Build history of the part. All positions in model axes, mm. Face numbers are marked on the shaded views. A direction names the side the tool comes from. Round coordinates to 2 decimals unless told otherwise and drop trailing zeros. Write each loop counter-clockwise with the first axis right and the second up, starting at its lowest first coordinate (ties: lowest second). Pieces come first, ordered by that corner, then holes. Notation, with made-up numbers: (66, -6.75) -> (108, -6.75) arc R35 ccw to (108, 25.25) -> close; hole circle Ø9 at (81.25, 65). An arc over 180 degrees is marked (long way). Answer as CSV lines item,"result".
from build123d import *

# Parameters (mm, degrees)
SKETCH1_W           = 33
SKETCH1_H           = 33
SKETCH1_R           = 1.5
BOSS_EXTRUDE1_DEPTH = 2.5
FILLET1_R           = 5
SKETCH2_W           = 15
SKETCH2_H           = 5.6
SKETCH2_W_2         = 5.6
SKETCH2_H_2         = 15
BOSS_EXTRUDE2_DEPTH = 7
SKETCH3_W           = 12
SKETCH3_H           = 11
BOSS_EXTRUDE3_DEPTH = 4


with BuildPart() as part:
    # Sketch1 → Boss-Extrude1 (new body)
    with BuildSketch(Plane.XY):
        with Locations((-3.4417913, -5.340458015)):
            Rectangle(SKETCH1_W, SKETCH1_H)
        with Locations((-15.4417913, 6.659541985)):
            Circle(SKETCH1_R, mode=Mode.SUBTRACT)
        with Locations(Location((8.5582087, 6.659541985, 0), (0, 0, 180))):
            Circle(SKETCH1_R, mode=Mode.SUBTRACT)
        with Locations(Location((-15.4417913, -17.340458015, 0), (0, 0, 180))):
            Circle(SKETCH1_R, mode=Mode.SUBTRACT)
        with Locations((8.5582087, -17.340458015)):
            Circle(SKETCH1_R, mode=Mode.SUBTRACT)
        with Locations((-10.5917913, -12.940458015)):
            Circle(SKETCH1_R, mode=Mode.SUBTRACT)
        with Locations(Location((3.7082087, -12.940458015, 0), (0, 0, 180))):
            Circle(SKETCH1_R, mode=Mode.SUBTRACT)
        with Locations(Location((-10.5917913, 2.259541985, 0), (0, 0, 180))):
            Circle(SKETCH1_R, mode=Mode.SUBTRACT)
        with Locations((3.7082087, 2.259541985)):
            Circle(SKETCH1_R, mode=Mode.SUBTRACT)
    extrude(amount=BOSS_EXTRUDE1_DEPTH)

    # Fillet1
    fillet1_edges = [part.edges().sort_by_distance(p)[0] for p in [
        (-19.9417913, 11.159541985, 1.25),
        (13.0582087, 11.159541985, 1.25),
        (13.0582087, -21.840458015, 1.25),
        (-19.9417913, -21.840458015, 1.25),
    ]]
    fillet(fillet1_edges, radius=FILLET1_R)

    # Sketch2 → Boss-Extrude2 (add)
    with BuildSketch(Plane.XY.offset(2.5)):
        with Locations((-3.4417913, -19.040458015)):
            Rectangle(SKETCH2_W, SKETCH2_H)
        with Locations((11.2582087, -5.340458015)):
            Rectangle(SKETCH2_W_2, SKETCH2_H_2)
    extrude(amount=BOSS_EXTRUDE2_DEPTH)

    # Sketch3 → Boss-Extrude3 (add)
    with BuildSketch(Plane.XY.offset(2.5)):
        with Locations((-3.4417913, -5.340458015)):
            Rectangle(SKETCH3_W, SKETCH3_H)
    extrude(amount=BOSS_EXTRUDE3_DEPTH)


solid = part.part
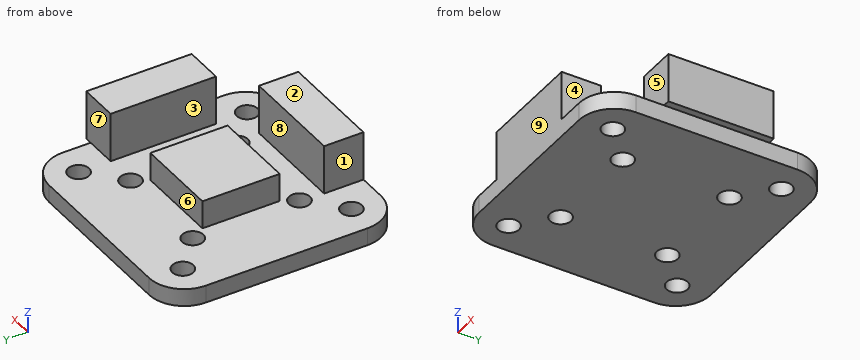
1. Mould opens along X. For the marked faces 1, 2, 3 and 4 say: +X half, -X half, draft (parallel to the pull), parting line (faces both ways), or undercut.
Results found:
face 1,"-X half"
face 2,"draft"
face 3,"undercut"
face 4,"+X half"
2. Which spindle directions (+Z, -Z, +X, -X, +Y, -Y) get a long thin tool onto all of the face, cutting with end or side? Do the marked faces 5, 6, 7, 8 and 9. Say none if no direction does.
Results found:
face 5,"+Z, +X, -X, -Y"
face 6,"+Z, -X, +Y"
face 7,"+Z, +X, -X, +Y"
face 8,"+Z, +X, -X"
face 9,"+Z, -Z, +X, -X, -Y"
3. Cut at A-A, the plane z = 7. Write the cut outline in (x, y).
Results found:
outline,"(-10.94, -21.84) -> (4.06, -21.84) -> (4.06, -16.24) -> (-10.94, -16.24) -> close; (8.46, -12.84) -> (14.06, -12.84) -> (14.06, 2.16) -> (8.46, 2.16) -> close"
4. Cut at C-C, the plane y = -14. Write the cut outline in (x, z).
Results found:
outline,"(-19.94, 0) -> (-11.65, 0) -> (-11.65, 2.5) -> (-19.94, 2.5) -> close; (-9.53, 0) -> (2.65, 0) -> (2.65, 2.5) -> (-9.53, 2.5) -> close; (4.77, 0) -> (13.06, 0) -> (13.06, 2.5) -> (4.77, 2.5) -> close"
5. Probe line 1 along X through (y, z) = (-7, 4); line 2 along Y through (x, z) = (-16, 2); line 3 along Y through (x, z) = (1, 5). List the from-to ranges inside material, lowest first.
Results found:
line 1,"x = -9.44 to 2.56, 8.46 to 14.06"
line 2,"y = -21.73 to -18.73, -15.95 to 5.27, 8.05 to 11.05"
line 3,"y = -21.84 to -16.24, -10.84 to 0.16"
6. Cut at B-B, the plane x = -10. Write the cut outline in (y, z).
Results found:
outline,"(-21.84, 0) -> (-14.32, 0) -> (-14.32, 2.5) -> (-16.24, 2.5) -> (-16.24, 9.5) -> (-21.84, 9.5) -> close; (-11.56, 0) -> (0.88, 0) -> (0.88, 2.5) -> (-11.56, 2.5) -> close; (3.64, 0) -> (11.16, 0) -> (11.16, 2.5) -> (3.64, 2.5) -> close"
7. Cut at D-D, the plane x = -4. Write the cut outline in (y, z).
Results found:
outline,"(-21.84, 0) -> (11.16, 0) -> (11.16, 2.5) -> (0.16, 2.5) -> (0.16, 6.5) -> (-10.84, 6.5) -> (-10.84, 2.5) -> (-16.24, 2.5) -> (-16.24, 9.5) -> (-21.84, 9.5) -> close"
8. Drop flat-ended pins along their axis: pin 1 Ø3 at (y, z) = (-19.5, 4.5) entering from +X; pin 2 Ø3 at (x, z) = (2.5, 5.5) entering from +Y; pin 3 Ø1.5 at (x, y) = (0.5, 5) entering from -Z; pin 4 Ø2.5 at (x, y) = (-10.59, 2.26) entering from +Z. Give the stop position or say it passes through.
Results found:
pin 1,"stops at x = 4.06"
pin 2,"stops at y = 0.16"
pin 3,"stops at z = 0"
pin 4,"passes through"
